from build123d import *

# Parameters (mm, degrees)
SKETCH1_R           = 1.6
BOSS_EXTRUDE1_DEPTH = 10
CUT_EXTRUDE1_DEPTH  = 8.5
SKETCH3_R           = 2.8
CUT_EXTRUDE2_DEPTH  = 8
FILLET1_R           = 3
FILLET2_R           = 3
FILLET3_R           = 0.75
CUT_EXTRUDE3_DEPTH  = 0.5


with BuildPart() as part:
    # Sketch1 → Boss-Extrude1 (new body)
    with BuildSketch(Plane(origin=(0, 0, 0), x_dir=(1, 0, 0), z_dir=(0, 1, 0))):
        with BuildLine():
            ThreePointArc((12, -16), (14.828427125, -14.828427125), (16, -12))
            Line((16, -12), (16, 12))
            ThreePointArc((16, 12), (14.828427125, 14.828427125), (12, 16))
            Line((12, 16), (-12, 16))
            ThreePointArc((-12, 16), (-14.828427125, 14.828427125), (-16, 12))
            Line((-16, 12), (-16, -12))
            ThreePointArc((-16, -12), (-14.828427125, -14.828427125), (-12, -16))
            Line((-12, -16), (12, -16))
        make_face()
        with Locations((-12, -12)):
            Circle(SKETCH1_R, mode=Mode.SUBTRACT)
        with Locations((12, -12)):
            Circle(SKETCH1_R, mode=Mode.SUBTRACT)
        with Locations((-12, 12)):
            Circle(SKETCH1_R, mode=Mode.SUBTRACT)
        with Locations((12, 12)):
            Circle(SKETCH1_R, mode=Mode.SUBTRACT)
    extrude(amount=BOSS_EXTRUDE1_DEPTH)

    # Sketch2 → Cut-Extrude1 (cut)
    with BuildSketch(Plane.XZ):
        with BuildLine():
            Line((-8, -16), (8, -16))
            Line((8, -16), (8, -11.489125293))
            ThreePointArc((8, -11.489125293), (0, 14), (-8, -11.489125293))
            Line((-8, -11.489125293), (-8, -16))
        make_face()
    extrude(amount=-CUT_EXTRUDE1_DEPTH, mode=Mode.SUBTRACT)

    # Sketch3 → Cut-Extrude2 (cut)
    with BuildSketch(Plane(origin=(0, 10, 0), x_dir=(1, 0, 0), z_dir=(0, 1, 0))):
        with Locations((-12, 12)):
            Circle(SKETCH3_R)
        with Locations((12, 12)):
            Circle(SKETCH3_R)
        with Locations((12, -12)):
            Circle(SKETCH3_R)
        with Locations((-12, -12)):
            Circle(SKETCH3_R)
    extrude(amount=-CUT_EXTRUDE2_DEPTH, mode=Mode.SUBTRACT)

    # Fillet1
    fillet1_edges = [part.edges().sort_by_distance(p)[0] for p in [
        (8, 4.25, -11.489125293),
        (-8, 4.25, -11.489125293),
    ]]
    fillet(fillet1_edges, radius=FILLET1_R)

    # Fillet2
    fillet2_edges = [part.edges().sort_by_distance(p)[0] for p in [
        (8, 8.5, -14.480740698),
        (-8, 8.5, -14.480740698),
        (0, 8.5, 14),
        (-8.277544361, 8.5, -11.701229321),
        (8.277544361, 8.5, -11.701229321),
    ]]
    fillet(fillet2_edges, radius=FILLET2_R)

    # Fillet3
    fillet3_edges = [part.edges().sort_by_distance(p)[0] for p in [
        (0, 10, 16),
        (14.828427125, 10, 14.828427125),
        (16, 10, 0),
        (14.828427125, 10, -14.828427125),
        (0, 10, -16),
        (-14.828427125, 10, -14.828427125),
        (-16, 10, 0),
        (-14.828427125, 10, 14.828427125),
    ]]
    fillet(fillet3_edges, radius=FILLET3_R)

    # Sketch6 → Cut-Extrude3 (cut)
    with BuildSketch(Plane(origin=(0, 10, 0), x_dir=(1, 0, 0), z_dir=(0, 1, 0))):
        Polygon((-6.741615885, -7.094845439), (-4.074949219, -4.428178772), (-6.741615885, -4.428178772), (-9.408282552, -7.094845439), align=None)
        Polygon((-2.741615885, -4.428178772), (-4.074949219, -4.428178772), (-6.741615885, -7.094845439), (-5.408282552, -7.094845439), align=None)
        Polygon((1.258384115, -7.094845439), (3.925050781, -4.428178772), (-0.074949219, -4.428178772), (-2.741615885, -7.094845439), align=None)
        Polygon((3.925050781, -4.428178772), (6.591717448, -1.761512106), (2.591717448, -1.761512106), (-0.074949219, -4.428178772), align=None)
        Polygon((6.591717448, 0.905154561), (5.258384115, 0.905154561), (2.591717448, -1.761512106), (6.591717448, -1.761512106), align=None)
        Polygon((2.591717448, -1.761512106), (5.258384115, 0.905154561), (1.258384115, 0.905154561), (-1.408282552, -1.761512106), align=None)
        Polygon((-1.408282552, -1.761512106), (1.258384115, 0.905154561), (-2.741615885, 0.905154561), (-5.408282552, -1.761512106), align=None)
        Polygon((-5.408282552, -1.761512106), (-2.741615885, 0.905154561), (-6.741615885, 0.905154561), (-6.741615885, -1.761512106), align=None)
        Polygon((-2.741615885, 0.905154561), (-0.074949219, 3.571821228), (-4.074949219, 3.571821228), (-6.741615885, 0.905154561), align=None)
        Polygon((-0.074949219, 3.571821228), (2.591717448, 6.238487894), (-1.408282552, 6.238487894), (-4.074949219, 3.571821228), align=None)
        Polygon((3.925050781, 3.571821228), (6.591717448, 6.238487894), (2.591717448, 6.238487894), (-0.074949219, 3.571821228), align=None)
        Polygon((5.258384115, 3.571821228), (7.925050781, 6.238487894), (6.591717448, 6.238487894), (3.925050781, 3.571821228), align=None)
    extrude(amount=-CUT_EXTRUDE3_DEPTH, mode=Mode.SUBTRACT)


solid = part.part
Verification items for the finished model (mm, model axes). A direction names the side the tool comes from. Coordinates: 2 decimals unless noted, no trailing zeros. Order: outer loops, then holes, each group sorted by start corner. A loop starts at its lowest first (then second) coordinate and runs counter-clockwise, first axis right, second up. Notation, with made-up numbers: M 78,37.25 L 136,37.25 A31 ccw 136,69.25 Z; hole C -30,-34.5 d9. An arc over 180 degrees is marked long. One line per item, written item: value. Start each with the question number.
Item 1: Access from +Z, -Z, +X, -X, +Y, -Y to the whole of each face (thin tool, end or side, straight path). Record for faces 1 (the flat face through (-4.094, 9.754, 5.78)), 2 (the cylindrical face through (-7.14, 7.6, -14.5)), 3 (the cylindrical face through (10.4, 0.99, -12.07)), 4 (the cylindrical face through (-8.27, 2.79, -11.72)).
Item 2: Gauge pin test, flat ends, axial feed: pin 1 (10 mm diameter, centred on x = -4.5, z = 11, fed in from -Y); pin 2 (1 mm diameter, centred on x = -10, z = 11, fed in from +Y); pin 3 (3.5 mm diameter, centred on y = 2.5, z = -14, fed in from +X); pin 4 (2.5 mm diameter, centred on x = 12, z = 12, fed in from +Y). Record the tip position at first contact, or that the pin passes through.
Item 3: Sectioned sample at B-B (y = 7). Enter the section's corners in (x, z), then the cut area to 3 significant figures.
Item 4: Scan lines: probe 1 along Z at (x, y) = (-12, 5); probe 2 along X at (y, z) = (6.75, 11); probe 3 along X at (y, z) = (7.75, -9.5). Record each from-to range of solid material in increasing order.
Item 5: Sectioned sample at A-A (y = 3). Enter the section's corners in (x, z).
Item 6: Mould release check, pull along X, two halves, no side actions. Record for faces 5 (the flat face through (3, 9, -16)), 6 (the cylindrical face through (-14.859, 4.56, 14.797)), 7 (the cylindrical face through (14.586, 6.056, 13.072)): released by +X, released by -X, zero draft, split by the parting line, or undercut.
Conclusion:
1. face 1: +Y
1. face 2: -Z, -Y
1. face 3: +Y, -Y
1. face 4: -Y
2. pin 1: stops at y = 0
2. pin 2: stops at y = 2
2. pin 3: stops at x = 15.99
2. pin 4: passes through
3. outline: M -16,-12 A4 ccw -12,-16 L -7.6,-16 L -7.6,-12.96 A3.4 ccw -8.8,-10.37 A13.6 cw long 8.8,-10.37 A3.4 ccw 7.6,-12.96 L 7.6,-16 L 12,-16 A4 ccw 16,-12 L 16,12 A4 ccw 12,16 L -12,16 A4 ccw -16,12 Z; hole C -12,-12 d5.6; hole C -12,12 d5.6; hole C 12,-12 d5.6; hole C 12,12 d5.6
3. area: 282 mm^2
4. probe 1: z = -16 to -14.8, -9.2 to -7.21, 7.21 to 9.2, 14.8 to 16
4. probe 2: x = -16 to -14.62, -9.38 to -8.21, 8.21 to 9.38, 14.62 to 16
4. probe 3: x = -16 to -13.26, -10.74 to -8.85, 8.85 to 10.74, 13.26 to 16
5. outline: M -16,-12 A4 ccw -12,-16 L -8,-16 L -8,-12.96 A3 ccw -9.06,-10.67 A14 cw long 9.06,-10.67 A3 ccw 8,-12.96 L 8,-16 L 12,-16 A4 ccw 16,-12 L 16,12 A4 ccw 12,16 L -12,16 A4 ccw -16,12 Z; hole C -12,-12 d5.6; hole C -12,12 d5.6; hole C 12,-12 d5.6; hole C 12,12 d5.6
6. face 5: zero draft
6. face 6: released by -X
6. face 7: undercut
